Model file for the job. Use its own axes, mm. A direction names the side the tool comes from. Give positions to 0.01 mm unless a question says otherwise; leave off trailing zeros. Order: outer loops, then holes, each group sorted by start corner. A loop starts at its lowest first (then second) coordinate and runs counter-clockwise, first axis right, second up. Notation, with made-up numbers: (38.25, -27.5) -> (74.25, -27.5) arc R16 cw to (74.25, -1.5) -> close; hole circle Ø11 at (-31, 59.5). An arc over 180 degrees is marked (long way). Use CSV: the item, a comma, the result in double quotes. Start each with the question number.
1. Pull direction Y, two halves, no side cores. Call faces 1 (the flat face through (4, -25, 0)), 2 (the cylindrical face through (-2.24, -40.5, 4.56)): released by +Y, released by -Y, zero draft, split by the parting line, or undercut.
2. Cut at A-A on y = -24. List the corners of the cut face in (x, z), then the cut area to 3 significant figures.
3. Cut at B-B on z = 12. List the corners of the cut face in (x, y), then the cut area to 3 significant figures.
4. Cut at D-D on y = -31. List the corners of the cut face in (x, z).
5. Cut at C-C on x = 4. List the corners of the cut face in (y, z), then the cut area to 3 significant figures.
6. Drop flat-ended pins along their axis: pin 1 (4.5 mm diameter, centred on y = -11.5, z = 5, fed in from +X); pin 2 (1.8 mm diameter, centred on y = -19, z = 16, fed in from -X). Give the stop position or say it passes through.
7. Wall check: line 1 (Y direction, x = 8.75, z = 45); line 2 (Z direction, x = 9, y = 0); line 3 (Y direction, x = -0.5, z = 47). Give the ranges that are in metal, low to high. Write a range as from..to.
8. 3-axis set-ups, long thin cutter, end or side, ignore diameter. For faces 3 (the flat face through (-2, 5, 42)), 4 (the flat face through (10, -21.032, 26)), 5 (the cylindrical face through (-2.27, 3.96, 7.97)): which of +Z, -Z, +X, -X, +Y, -Y reach the whole face in a straight line?
```python
from build123d import *

# Parameters (mm, degrees)
SKETCH_1_W          = 13.5
SKETCH_1_H          = 67.5
EXTRUDE_1_DEPTH     = 52
CUT_EXTRUDE_1_REACH = 81.819
SKETCH_2_W          = 48
SKETCH_2_H          = 63.5
EXTRUDE_2_REACH     = 80.099
SKETCH_3_W          = 2
SKETCH_3_H          = 6
SKETCH_9_W          = 2
SKETCH_9_H          = 4
EXTRUDE_3_DEPTH     = 4
SKETCH_10_W         = 2
SKETCH_10_H         = 4
EXTRUDE_4_DEPTH     = 4
SKETCH_11_W         = 2
SKETCH_11_H         = 4
EXTRUDE_5_DEPTH     = 4
SKETCH_12_W         = 2
SKETCH_12_H         = 4
EXTRUDE_6_DEPTH     = 4
FILLET_1_R          = 4


with BuildPart() as part:
    # 草图1 → 凸台-拉伸1 (new body)
    with BuildSketch(Plane.XY):
        with Locations((3.959815951, -25.281820368)):
            Rectangle(SKETCH_1_W, SKETCH_1_H)
    extrude(amount=EXTRUDE_1_DEPTH)

    # 草图2 → 切除-拉伸1 (cut, up to next)
    with BuildSketch(Plane(origin=(10.709815951, 0, 0), x_dir=(0, 0, -1), z_dir=(1, 0, 0)), mode=Mode.PRIVATE) as cut_extrude_1_sk1:
        with Locations((-26, -25.281820368)):
            Rectangle(SKETCH_2_W, SKETCH_2_H)
    cut_extrude_1_tool1 = extrude(cut_extrude_1_sk1.sketch, amount=-CUT_EXTRUDE_1_REACH, mode=Mode.PRIVATE) & part.part
    add(cut_extrude_1_tool1.solids().sort_by_distance((10.709816, -25.28182, 26))[0], mode=Mode.SUBTRACT)

    # 草图3 → 凸台-拉伸2 (add, up to next)
    with BuildSketch(Plane(origin=(0, 0, 50), x_dir=(-1, 0, 0), z_dir=(0, 0, -1)), mode=Mode.PRIVATE) as extrude_2_sk1:
        with Locations((-9.709815951, -4.031820368)):
            Rectangle(SKETCH_3_W, SKETCH_3_H)
    extrude_2_tool1 = extrude(extrude_2_sk1.sketch, amount=EXTRUDE_2_REACH, mode=Mode.PRIVATE) - part.part
    # 草图3 → 凸台-拉伸2 (add, up to next)
    with BuildSketch(Plane(origin=(0, 0, 50), x_dir=(-1, 0, 0), z_dir=(0, 0, -1)), mode=Mode.PRIVATE) as extrude_2_sk2:
        with Locations((-9.709815951, -18.031820368)):
            Rectangle(SKETCH_3_W, SKETCH_3_H)
    extrude_2_tool2 = extrude(extrude_2_sk2.sketch, amount=EXTRUDE_2_REACH, mode=Mode.PRIVATE) - part.part
    # 草图3 → 凸台-拉伸2 (add, up to next)
    with BuildSketch(Plane(origin=(0, 0, 50), x_dir=(-1, 0, 0), z_dir=(0, 0, -1)), mode=Mode.PRIVATE) as extrude_2_sk3:
        with Locations((-9.709815951, -32.031820368)):
            Rectangle(SKETCH_3_W, SKETCH_3_H)
    extrude_2_tool3 = extrude(extrude_2_sk3.sketch, amount=EXTRUDE_2_REACH, mode=Mode.PRIVATE) - part.part
    # 草图3 → 凸台-拉伸2 (add, up to next)
    with BuildSketch(Plane(origin=(0, 0, 50), x_dir=(-1, 0, 0), z_dir=(0, 0, -1)), mode=Mode.PRIVATE) as extrude_2_sk4:
        with Locations((-9.709815951, -46.031820368)):
            Rectangle(SKETCH_3_W, SKETCH_3_H)
    extrude_2_tool4 = extrude(extrude_2_sk4.sketch, amount=EXTRUDE_2_REACH, mode=Mode.PRIVATE) - part.part
    add(extrude_2_tool1.solids().sort_by_distance((9.709816, -4.03182, 50))[0])
    add(extrude_2_tool2.solids().sort_by_distance((9.709816, -18.03182, 50))[0])
    add(extrude_2_tool3.solids().sort_by_distance((9.709816, -32.03182, 50))[0])
    add(extrude_2_tool4.solids().sort_by_distance((9.709816, -46.03182, 50))[0])

    # 草图9 → 凸台-拉伸3 (add)
    with BuildSketch(Plane(origin=(0, 0, 50), x_dir=(-1, 0, 0), z_dir=(0, 0, -1))):
        with Locations((1.790184049, -0.531820368)):
            Rectangle(SKETCH_9_W, SKETCH_9_H)
        with Locations((1.790184049, -10.531820368)):
            Rectangle(SKETCH_9_W, SKETCH_9_H)
        with Locations((1.790184049, -20.531820368)):
            Rectangle(SKETCH_9_W, SKETCH_9_H)
        with Locations((1.790184049, -30.531820368)):
            Rectangle(SKETCH_9_W, SKETCH_9_H)
        with Locations((1.790184049, -40.531820368)):
            Rectangle(SKETCH_9_W, SKETCH_9_H)
        with Locations((1.790184049, -50.531820368)):
            Rectangle(SKETCH_9_W, SKETCH_9_H)
    extrude(amount=EXTRUDE_3_DEPTH)

    # 草图10 → 凸台-拉伸4 (add)
    with BuildSketch(Plane.XZ.offset(-6.468179632)):
        with Locations((-1.790184049, 8)):
            Rectangle(SKETCH_10_W, SKETCH_10_H)
        with Locations((-1.790184049, 17)):
            Rectangle(SKETCH_10_W, SKETCH_10_H)
        with Locations((-1.790184049, 26)):
            Rectangle(SKETCH_10_W, SKETCH_10_H)
        with Locations((-1.790184049, 35)):
            Rectangle(SKETCH_10_W, SKETCH_10_H)
        with Locations((-1.790184049, 44)):
            Rectangle(SKETCH_10_W, SKETCH_10_H)
    extrude(amount=EXTRUDE_4_DEPTH)

    # 草图11 → 凸台-拉伸5 (add)
    with BuildSketch(Plane(origin=(0, -57.031820368, 0), x_dir=(1, 0, 0), z_dir=(0, 1, 0))):
        with Locations((-1.790184049, -44)):
            Rectangle(SKETCH_11_W, SKETCH_11_H)
        with Locations((-1.790184049, -35)):
            Rectangle(SKETCH_11_W, SKETCH_11_H)
        with Locations((-1.790184049, -26)):
            Rectangle(SKETCH_11_W, SKETCH_11_H)
        with Locations((-1.790184049, -17)):
            Rectangle(SKETCH_11_W, SKETCH_11_H)
        with Locations((-1.790184049, -8)):
            Rectangle(SKETCH_11_W, SKETCH_11_H)
    extrude(amount=EXTRUDE_5_DEPTH)

    # 草图12 → 凸台-拉伸6 (add)
    with BuildSketch(Plane.XY.offset(2)):
        with Locations((-1.790184049, -0.531820368)):
            Rectangle(SKETCH_12_W, SKETCH_12_H)
        with Locations((-1.790184049, -10.531820368)):
            Rectangle(SKETCH_12_W, SKETCH_12_H)
        with Locations((-1.790184049, -20.531820368)):
            Rectangle(SKETCH_12_W, SKETCH_12_H)
        with Locations((-1.790184049, -30.531820368)):
            Rectangle(SKETCH_12_W, SKETCH_12_H)
        with Locations((-1.790184049, -40.531820368)):
            Rectangle(SKETCH_12_W, SKETCH_12_H)
        with Locations((-1.790184049, -50.531820368)):
            Rectangle(SKETCH_12_W, SKETCH_12_H)
    extrude(amount=EXTRUDE_6_DEPTH)

    # 圆角1
    # the kernel refuses this fillet: 4 mm, written as the material it takes off along each edge
    with BuildSketch(Plane(origin=(-2.790184049, -39.871566331, 46), x_dir=(0, 0, 1), z_dir=(0, -1, 0))) as fillet_1_piece_1_section:
        with BuildLine():
            CenterArc((3.464101615, -4), FILLET_1_R, 90, 60)
            Line((0, -2), (0, 0))
            Line((0, 0), (3.464101615, 0))
        make_face()
    fillet_1_piece_1 = extrude(amount=21.320508076, mode=Mode.PRIVATE)
    fillet_1_piece_1 = split(fillet_1_piece_1, bisect_by=Plane(origin=(-2.261213867, -53.031820368, 47.460101615), z_dir=(0, 1, 0)), keep=Keep.TOP, mode=Mode.PRIVATE)
    add(fillet_1_piece_1, mode=Mode.SUBTRACT)
    with BuildSketch(Plane(origin=(-2.790184049, -53.031820368, 46), x_dir=(0, -1, 0), z_dir=(0, 0, -1)), Plane(origin=(-2.790184049, -11.192074406, 6), x_dir=(0, 0, -1), z_dir=(0, 1, 0)), Plane(origin=(-2.790184049, 2.468179632, 6), x_dir=(0, 1, 0), z_dir=(0, 0, 1))) as fillet_1_piece_2:
        with BuildLine():
            CenterArc((3.464101615, -4), FILLET_1_R, 90, 60)
            Line((0, -2), (0, 0))
            Line((0, 0), (3.464101615, 0))
        make_face()
    extrude(amount=12.660254038, mode=Mode.SUBTRACT)
    with BuildSketch(Plane(origin=(-2.790184049, -29.871566331, 46), x_dir=(0, 0, 1), z_dir=(0, -1, 0)), Plane(origin=(-2.790184049, -19.871566331, 46), x_dir=(0, 0, 1), z_dir=(0, -1, 0)), Plane(origin=(-2.790184049, 0.128433669, 46), x_dir=(0, 0, 1), z_dir=(0, -1, 0)), Plane(origin=(-2.790184049, -9.871566331, 46), x_dir=(0, 0, 1), z_dir=(0, -1, 0))) as fillet_1_piece_3:
        with BuildLine():
            CenterArc((3.464101615, -4), FILLET_1_R, 90, 60)
            Line((0, -2), (0, 0))
            Line((0, 0), (3.464101615, 0))
        make_face()
    extrude(amount=21.320508076, mode=Mode.SUBTRACT)
    with BuildSketch(Plane(origin=(-2.790184049, -53.031820368, 24.339745962), x_dir=(0, -1, 0), z_dir=(0, 0, 1)), Plane(origin=(-2.790184049, -53.031820368, 15.339745962), x_dir=(0, -1, 0), z_dir=(0, 0, 1)), Plane(origin=(-2.790184049, -53.031820368, 6.339745962), x_dir=(0, -1, 0), z_dir=(0, 0, 1)), Plane(origin=(-2.790184049, -29.871566331, 6), x_dir=(0, 0, -1), z_dir=(0, -1, 0)), Plane(origin=(-2.790184049, -9.871566331, 6), x_dir=(0, 0, -1), z_dir=(0, -1, 0)), Plane(origin=(-2.790184049, -19.871566331, 6), x_dir=(0, 0, -1), z_dir=(0, -1, 0)), Plane(origin=(-2.790184049, 0.128433669, 6), x_dir=(0, 0, -1), z_dir=(0, -1, 0)), Plane(origin=(-2.790184049, 2.468179632, 27.660254038), x_dir=(0, 1, 0), z_dir=(0, 0, -1)), Plane(origin=(-2.790184049, 2.468179632, 36.660254038), x_dir=(0, 1, 0), z_dir=(0, 0, -1)), Plane(origin=(-2.790184049, 2.468179632, 45.660254038), x_dir=(0, 1, 0), z_dir=(0, 0, -1))) as fillet_1_piece_4:
        with BuildLine():
            CenterArc((3.464101615, 4), FILLET_1_R, 210, 60)
            Line((0, 2), (0, 0))
            Line((0, 0), (3.464101615, 0))
        make_face()
    extrude(amount=21.320508076, mode=Mode.SUBTRACT)
    with BuildSketch(Plane(origin=(-2.790184049, -39.871566331, 6), x_dir=(0, 0, -1), z_dir=(0, -1, 0)), Plane(origin=(-2.790184049, 2.468179632, 46), x_dir=(0, 1, 0), z_dir=(0, 0, -1))) as fillet_1_piece_5:
        with BuildLine():
            CenterArc((3.464101615, 4), FILLET_1_R, 210, 60)
            Line((0, 2), (0, 0))
            Line((0, 0), (3.464101615, 0))
        make_face()
    extrude(amount=12.660254038, mode=Mode.SUBTRACT)
    with BuildSketch(Plane(origin=(-2.790184049, -53.031820368, -2.660254038), x_dir=(0, -1, 0), z_dir=(0, 0, 1))) as fillet_1_piece_6_section:
        with BuildLine():
            CenterArc((3.464101615, 4), FILLET_1_R, 210, 60)
            Line((0, 2), (0, 0))
            Line((0, 0), (3.464101615, 0))
        make_face()
    fillet_1_piece_6 = extrude(amount=21.320508076, mode=Mode.PRIVATE)
    fillet_1_piece_6 = split(fillet_1_piece_6, bisect_by=Plane(origin=(-2.261213867, -54.491921984, 2), z_dir=(0, 0, 1)), keep=Keep.TOP, mode=Mode.PRIVATE)
    add(fillet_1_piece_6, mode=Mode.SUBTRACT)
    with BuildSketch(Plane(origin=(-2.790184049, -11.192074406, 46), x_dir=(0, 0, 1), z_dir=(0, 1, 0))) as fillet_1_piece_7_section:
        with BuildLine():
            CenterArc((3.464101615, 4), FILLET_1_R, 210, 60)
            Line((0, 2), (0, 0))
            Line((0, 0), (3.464101615, 0))
        make_face()
    fillet_1_piece_7 = extrude(amount=21.320508076, mode=Mode.PRIVATE)
    fillet_1_piece_7 = split(fillet_1_piece_7, bisect_by=Plane(origin=(-2.261213867, 2.468179632, 47.460101615), z_dir=(0, -1, 0)), keep=Keep.TOP, mode=Mode.PRIVATE)
    add(fillet_1_piece_7, mode=Mode.SUBTRACT)


solid = part.part
```
Verdict:
1,face 1,"zero draft"
1,face 2,"undercut"
2,outline,"(-2.79, 0) -> (10.71, 0) -> (10.71, 2) -> (-2.79, 2) -> close; (-2.79, 50) -> (10.71, 50) -> (10.71, 52) -> (-2.79, 52) -> close"
2,area,"54.0 mm^2"
3,outline,"(-2.79, -59.03) -> (10.71, -59.03) -> (10.71, -57.03) -> (-2.79, -57.03) -> close; (-2.79, 6.47) -> (10.71, 6.47) -> (10.71, 8.47) -> (-2.79, 8.47) -> close; (8.71, -49.03) -> (10.71, -49.03) -> (10.71, -43.03) -> (8.71, -43.03) -> close; (8.71, -35.03) -> (10.71, -35.03) -> (10.71, -29.03) -> (8.71, -29.03) -> close; (8.71, -21.03) -> (10.71, -21.03) -> (10.71, -15.03) -> (8.71, -15.03) -> close; (8.71, -7.03) -> (10.71, -7.03) -> (10.71, -1.03) -> (8.71, -1.03) -> close"
3,area,"102 mm^2"
4,outline,"(-2.79, 0) -> (10.71, 0) -> (10.71, 52) -> (-2.79, 52) -> (-2.79, 49.46) arc R4 ccw to (-0.79, 46) -> (-0.79, 50) -> (8.71, 50) -> (8.71, 2) -> (-0.79, 2) -> (-0.79, 6) arc R4 ccw to (-2.79, 2.54) -> close"
5,outline,"(-59.03, 0) -> (8.47, 0) -> (8.47, 52) -> (-59.03, 52) -> close; hole (-57.03, 2) -> (6.47, 2) -> (6.47, 50) -> (-57.03, 50) -> close"
5,area,"462 mm^2"
6,pin 1,"x = -0.79"
6,pin 2,"x = 8.71"
7,line 1,"-59.03..-57.03, -49.03..-43.03, -35.03..-29.03, -21.03..-15.03, -7.03..-1.03, 6.47..8.47"
7,line 2,"0..2, 50..52"
7,line 3,"-59.03..-57.03, 6.47..8.47"
8,face 3,"+X, -X"
8,face 4,"+X"
8,face 5,"-X"
